from build123d import *
from build123d.topology import SkipClean

# Parameters (mm, degrees)
SKETCH_1_W      = 33.865609136
SKETCH_1_H      = 190
SKETCH_1_R      = 2.65
EXTRUDE_1_DEPTH = 10
FILLET_1_R      = 10
EXTRUDE_2_DEPTH = 33.865609
FILLET_2_R      = 2


# Some blends are built 0.0001 mm under size
with BuildPart() as part:
    # 草图1 → 凸台-拉伸1 (new body)
    with BuildSketch(Plane.XY):
        Rectangle(SKETCH_1_W, SKETCH_1_H)
        with Locations((-6.85, 73)):
            Circle(SKETCH_1_R, mode=Mode.SUBTRACT)
        with Locations(Location((6.85, 73, 0), (0, 0, 180))):
            Circle(SKETCH_1_R, mode=Mode.SUBTRACT)
        with Locations(Location((-6.85, -73, 0), (0, 0, 180))):
            Circle(SKETCH_1_R, mode=Mode.SUBTRACT)
        with Locations((6.85, -73)):
            Circle(SKETCH_1_R, mode=Mode.SUBTRACT)
    extrude(amount=EXTRUDE_1_DEPTH)

    # 圆角1
    fillet_1_edges = [part.edges().sort_by_distance(p)[0] for p in [
        (0, -95, 10),
        (0, 95, 10),
    ]]
    fillet(fillet_1_edges, radius=FILLET_1_R - 0.0001)  # a hair under: the kernel refuses the full size

    # 草图2 → 凸台-拉伸2 (add, through all)
    with SkipClean():  # the faces are left unmerged after this step: merging them gives an invalid solid
        with BuildSketch(Plane.ZY.offset(16.932804568)):
            Polygon((44.6, 58.899086467), (10, 65), (10, 20), (44.6, 39.976319314), align=None)
            Polygon((44.6, -39.976319314), (10, -20), (10, -65), (44.6, -58.899086467), align=None)
        extrude(amount=-EXTRUDE_2_DEPTH)

    # 圆角2
    # the kernel refuses this fillet: 2 mm, written as the material it takes off along each edge
    with BuildSketch(Plane(origin=(16.932804568, -85.0001, 10), x_dir=(0, 0, -1), z_dir=(0, 1, 0))) as fillet_2_piece_1_section:
        with BuildLine():
            CenterArc((FILLET_2_R, FILLET_2_R), FILLET_2_R, 180, 90)
            Line((0, FILLET_2_R), (0, 0))
            Line((0, 0), (FILLET_2_R, 0))
        make_face()
    fillet_2_piece_1 = extrude(amount=25.0001, mode=Mode.PRIVATE)
    fillet_2_piece_1 = split(fillet_2_piece_1, bisect_by=Plane(origin=(16.479042192, -65.37988803, 7.84554792), z_dir=(0, -0.9848077530122075, 0.17364817766693394)), keep=Keep.TOP, mode=Mode.PRIVATE)
    add(fillet_2_piece_1, mode=Mode.SUBTRACT)
    with BuildSketch(Plane(origin=(-16.932804568, 85.0001, 10), x_dir=(0, 0, -1), z_dir=(0, -1, 0))) as fillet_2_piece_2_section:
        with BuildLine():
            CenterArc((FILLET_2_R, FILLET_2_R), FILLET_2_R, 180, 90)
            Line((0, FILLET_2_R), (0, 0))
            Line((0, 0), (FILLET_2_R, 0))
        make_face()
    fillet_2_piece_2 = extrude(amount=25.0001, mode=Mode.PRIVATE)
    fillet_2_piece_2 = split(fillet_2_piece_2, bisect_by=Plane(origin=(-16.479042192, 65.37988803, 7.84554792), z_dir=(0, 0.9848077530122075, 0.17364817766693394)), keep=Keep.TOP, mode=Mode.PRIVATE)
    add(fillet_2_piece_2, mode=Mode.SUBTRACT)
    with BuildSketch(Plane(origin=(16.932804568, 85.0001, 0.0001), x_dir=(0, 1, 0), z_dir=(0, 0, -1))) as fillet_2_piece_3:
        with BuildLine():
            CenterArc((9.9999 - FILLET_2_R, -FILLET_2_R), FILLET_2_R, 0, 90)
            Line((9.9999, -FILLET_2_R), (9.9999, 0))
            Line((9.9999, 0), (9.9999 - FILLET_2_R, 0))
        make_face()
    revolve(axis=Axis((16.932804568, 85.0001, 0.0001), (1, 0, 0)), revolution_arc=90, mode=Mode.SUBTRACT)
    with BuildSketch(Plane(origin=(16.932804568, -85.0001, 0.0001), x_dir=(0, -1, 0), z_dir=(0, 0, -1))) as fillet_2_piece_4:
        with BuildLine():
            CenterArc((9.9999 - FILLET_2_R, FILLET_2_R), FILLET_2_R, 270, 90)
            Line((9.9999 - FILLET_2_R, 0), (9.9999, 0))
            Line((9.9999, 0), (9.9999, FILLET_2_R))
        make_face()
    revolve(axis=Axis((16.932804568, -85.0001, 0.0001), (-1, 0, 0)), revolution_arc=90, mode=Mode.SUBTRACT)
    with BuildSketch(Plane(origin=(-16.932804568, 85.0001, 0.0001), x_dir=(0, 1, 0), z_dir=(0, 0, -1))) as fillet_2_piece_5:
        with BuildLine():
            CenterArc((9.9999 - FILLET_2_R, FILLET_2_R), FILLET_2_R, 270, 90)
            Line((9.9999, FILLET_2_R), (9.9999, 0))
            Line((9.9999, 0), (9.9999 - FILLET_2_R, 0))
        make_face()
    revolve(axis=Axis((-16.932804568, 85.0001, 0.0001), (1, 0, 0)), revolution_arc=90, mode=Mode.SUBTRACT)
    with BuildSketch(Plane(origin=(-16.932804568, -85.0001, 0.0001), x_dir=(0, -1, 0), z_dir=(0, 0, -1))) as fillet_2_piece_6:
        with BuildLine():
            CenterArc((9.9999 - FILLET_2_R, -FILLET_2_R), FILLET_2_R, 0, 90)
            Line((9.9999, -FILLET_2_R), (9.9999, 0))
            Line((9.9999, 0), (9.9999 - FILLET_2_R, 0))
        make_face()
    revolve(axis=Axis((-16.932804568, -85.0001, 0.0001), (-1, 0, 0)), revolution_arc=90, mode=Mode.SUBTRACT)
    with BuildSketch(Plane(origin=(16.932804568, 60, 10), x_dir=(0, 0, -1), z_dir=(0, 1, 0))) as fillet_2_piece_7_section:
        with BuildLine():
            CenterArc((FILLET_2_R, FILLET_2_R), FILLET_2_R, 180, 90)
            Line((0, FILLET_2_R), (0, 0))
            Line((0, 0), (FILLET_2_R, 0))
        make_face()
    fillet_2_piece_7 = extrude(amount=25.0001, mode=Mode.PRIVATE)
    fillet_2_piece_7 = split(fillet_2_piece_7, bisect_by=Plane(origin=(16.479042192, 65.37988803, 7.84554792), z_dir=(0, 0.9848077530122075, 0.17364817766693394)), keep=Keep.TOP, mode=Mode.PRIVATE)
    add(fillet_2_piece_7, mode=Mode.SUBTRACT)
    with BuildSketch(Plane(origin=(-19.819555914, 39.976319314, 44.6), x_dir=(0, -0.5000000000000052, -0.8660254037844355), z_dir=(1, 0, 0))) as fillet_2_piece_8:
        with BuildLine():
            CenterArc((FILLET_2_R * 0.57735026919, FILLET_2_R), FILLET_2_R, 210, 60)
            Line((-FILLET_2_R * 0.288675134595, FILLET_2_R * 0.5), (0, 0))
            Line((0, 0), (FILLET_2_R * 0.57735026919, 0))
        make_face()
    extrude(amount=39.639111692, mode=Mode.SUBTRACT)
    with BuildSketch(Plane(origin=(-16.932804568, 34.976319314, 44.6), x_dir=(0, 0, -1), z_dir=(0, 1, 0)), Plane(origin=(-16.932804568, -63.899086467, 44.6), x_dir=(0, 0, -1), z_dir=(0, 1, 0))) as fillet_2_piece_9:
        with BuildLine():
            CenterArc((FILLET_2_R, -FILLET_2_R), FILLET_2_R, 90, 90)
            Line((0, -FILLET_2_R), (0, 0))
            Line((0, 0), (FILLET_2_R, 0))
        make_face()
    extrude(amount=28.922767154, mode=Mode.SUBTRACT)
    with BuildSketch(Plane(origin=(-21.128302724, 58.899086467, 44.6), x_dir=(0, 0.17364817766693522, -0.9848077530122071), z_dir=(1, 0, 0))) as fillet_2_piece_10:
        with BuildLine():
            CenterArc((FILLET_2_R * 0.839099631177, -FILLET_2_R), FILLET_2_R, 90, 80)
            Line((-FILLET_2_R * 0.145708121835, -FILLET_2_R * 0.826351822333), (0, 0))
            Line((0, 0), (FILLET_2_R * 0.839099631177, 0))
        make_face()
    extrude(amount=42.256605312, mode=Mode.SUBTRACT)
    with BuildSketch(Plane(origin=(16.932804432, 34.976319314, 44.6), x_dir=(0, 0, -1), z_dir=(0, 1, 0)), Plane(origin=(16.932804432, -63.899086467, 44.6), x_dir=(0, 0, -1), z_dir=(0, 1, 0))) as fillet_2_piece_11:
        with BuildLine():
            CenterArc((FILLET_2_R, FILLET_2_R), FILLET_2_R, 180, 90)
            Line((0, FILLET_2_R), (0, 0))
            Line((0, 0), (FILLET_2_R, 0))
        make_face()
    extrude(amount=28.922767154, mode=Mode.SUBTRACT)
    with BuildSketch(Plane(origin=(-16.932804568, -60, 10), x_dir=(0, 0, -1), z_dir=(0, -1, 0))) as fillet_2_piece_12_section:
        with BuildLine():
            CenterArc((FILLET_2_R, FILLET_2_R), FILLET_2_R, 180, 90)
            Line((0, FILLET_2_R), (0, 0))
            Line((0, 0), (FILLET_2_R, 0))
        make_face()
    fillet_2_piece_12 = extrude(amount=25.0001, mode=Mode.PRIVATE)
    fillet_2_piece_12 = split(fillet_2_piece_12, bisect_by=Plane(origin=(-16.479042192, -65.37988803, 7.84554792), z_dir=(0, -0.9848077530122075, 0.17364817766693394)), keep=Keep.TOP, mode=Mode.PRIVATE)
    add(fillet_2_piece_12, mode=Mode.SUBTRACT)
    with BuildSketch(Plane(origin=(-19.819555914, -39.976319314, 44.6), x_dir=(0, 0.5000000000000052, -0.8660254037844355), z_dir=(1, 0, 0))) as fillet_2_piece_13:
        with BuildLine():
            CenterArc((FILLET_2_R * 0.57735026919, -FILLET_2_R), FILLET_2_R, 90, 60)
            Line((-FILLET_2_R * 0.288675134595, -FILLET_2_R * 0.5), (0, 0))
            Line((0, 0), (FILLET_2_R * 0.57735026919, 0))
        make_face()
    extrude(amount=39.639111692, mode=Mode.SUBTRACT)
    with BuildSketch(Plane(origin=(-21.128302724, -58.899086467, 44.6), x_dir=(0, -0.17364817766693183, -0.9848077530122078), z_dir=(1, 0, 0))) as fillet_2_piece_14:
        with BuildLine():
            CenterArc((FILLET_2_R * 0.839099631177, FILLET_2_R), FILLET_2_R, 190, 80)
            Line((-FILLET_2_R * 0.145708121835, FILLET_2_R * 0.826351822333), (0, 0))
            Line((0, 0), (FILLET_2_R * 0.839099631177, 0))
        make_face()
    extrude(amount=42.256605312, mode=Mode.SUBTRACT)
    with BuildSketch(Plane(origin=(-16.932804568, -95, -5), x_dir=(1, 0, 0), z_dir=(0, 0, 1)), Plane(origin=(-16.932804568, 95, -5), x_dir=(0, -1, 0), z_dir=(0, 0, 1))) as fillet_2_piece_15:
        with BuildLine():
            CenterArc((FILLET_2_R, FILLET_2_R), FILLET_2_R, 180, 90)
            Line((0, FILLET_2_R), (0, 0))
            Line((0, 0), (FILLET_2_R, 0))
        make_face()
    extrude(amount=5.0001, mode=Mode.SUBTRACT)
    with BuildSketch(Plane(origin=(16.932804568, -95, -5), x_dir=(-1, 0, 0), z_dir=(0, 0, 1)), Plane(origin=(16.932804568, 95, -5), x_dir=(0, -1, 0), z_dir=(0, 0, 1))) as fillet_2_piece_16:
        with BuildLine():
            CenterArc((FILLET_2_R, -FILLET_2_R), FILLET_2_R, 90, 90)
            Line((0, -FILLET_2_R), (0, 0))
            Line((0, 0), (FILLET_2_R, 0))
        make_face()
    extrude(amount=5.0001, mode=Mode.SUBTRACT)


solid = part.part
Could you check a few things on this model? Use its own coordinates, in mm. A direction names the side the tool comes from. Give positions to 0.01 mm unless a question says otherwise; leave off trailing zeros. Order: outer loops, then holes, each group sorted by start corner. A loop starts at its lowest first (then second) coordinate and runs counter-clockwise, first axis right, second up.
1. For pin 1 (8 mm diameter, centred on x = 4, z = 5.5, fed in from -Y); pin 2 (3 mm diameter, centred on x = -8, z = 6.5, fed in from +Y); pin 3 (6 mm diameter, centred on x = 5, y = -77, fed in from +Z); pin 4 (3 mm diameter, centred on x = 6.85, y = 73, fed in from +Z), each with a flat end and sliding along its axis, tell me the tip position at first contact or that it passes through.
Answers below:
pin 1: stops at y = -94.89
pin 2: stops at y = 93.66
pin 3: stops at z = 10
pin 4: passes through
2. Which directions (+Z, -Z, +X, -X, +Y, -Y) give clear straight access to the entire face, cutting with the end or side of a thin tool? Please do faces 5 (the flat face through (0, 75, 10)), 6 (the flat face through (0, 0, 10)), 7 (the flat face through (0, -75, 10)), 8 (the flat face through (0, 1, 0)).
Answers below:
face 5: +Z, +X, -X, +Y
face 6: +Z, +X, -X
face 7: +Z, +X, -X, -Y
face 8: -Z, +X, -X, +Y, -Y
3. Suppose I cut it at B-B (x = -6.85). State how many separate pieces and enclosed holes the cut face has, plus the area to 3 significant figures.
Answers below:
separate pieces: 3
enclosed holes: 0
area: 3,960 mm2
4. I need wall thicknesses on L1, parallel to Y at x = 6.85, z = 7.25; L2, parallel to Y at x = 6.85, z = 3; L3, parallel to Z at x = 7.5, y = 4. Which ranges of each line are inside material? Lowest first, please.
Answers below:
L1: y = -91.89 to -75.65, -70.35 to 70.35, 75.65 to 91.89
L2: y = -94.54 to -75.65, -70.35 to 70.35, 75.65 to 94.54
L3: z = 0 to 10
5. Thinking about a two-plate mould opening in X: for faces 1 (the cylindrical face through (-5.627, 70.649, 4.93)), 2 (the cylindrical face through (6.28, -75.59, 4.93)), 3 (the flat face through (0, -49, 44.6)), 4 (the flat face through (-16.933, -1, 7)), which applies, +X half, -X half, draft (parallel to the pull), parting line (faces both ways), or undercut?
Answers below:
face 1: undercut
face 2: undercut
face 3: draft
face 4: -X half
6. Suppose I cut it at C-C (z = 28). Write out the boundary of the cut face in (x, y), plus the area to 3 significant figures.
Answers below:
outline: (-16.93, -61.83) - (16.93, -61.83) - (16.93, -30.39) - (-16.93, -30.39) - close; (-16.93, 30.39) - (16.93, 30.39) - (16.93, 61.83) - (-16.93, 61.83) - close
area: 2,130 mm2
7. Suppose I cut it at A-A (y = 73). Write out the boundary of the cut face in (x, z).
Answers below:
outline: (-16.93, 0) - (-9.5, 0) - (-9.5, 10) - (-14.93, 10) arc R2 ccw to (-16.93, 8) - close; (-4.2, 0) - (4.2, 0) - (4.2, 10) - (-4.2, 10) - close; (9.5, 0) - (16.93, 0) - (16.93, 8) arc R2 ccw to (14.93, 10) - (9.5, 10) - close
